Verification items for the finished model (mm, model axes). A direction names the side the tool comes from. Coordinates: 2 decimals unless noted, no trailing zeros. Order: outer loops, then holes, each group sorted by start corner. A loop starts at its lowest first (then second) coordinate and runs counter-clockwise, first axis right, second up. Notation, with made-up numbers: (80.5, 71.25) -> (114.5, 71.25) arc R25 cw to (114.5, 100.25) -> close; hole circle Ø11 at (-5, 34). An arc over 180 degrees is marked (long way). Write item = value, one per line. Start each with the question number.
1. Cross-section at B-B on y = -14. Record the cut outline in (x, z), plus the area to 3 significant figures.
2. Set-up check for faces 5 (the flat face through (-28, 0, 4)), 6 (the flat face through (-40.846, -14.79, 22.722)), 7 (the cylindrical face through (-13.654, -14.79, 21.35)), 8 (the cylindrical face through (-38.355, -14.79, 10.279)), 9 (the flat face through (-13.237, -15, 8)): record each of +Z, -Z, +X, -X, +Y, -Y from which the full face is reachable in a straight line by a thin tool's end or side.
3. Cross-section at D-D on x = -25.5. Record the cut outline in (y, z), plus the area to 3 significant figures.
4. Cross-section at C-C on x = -19. Record the cut outline in (y, z).
5. Go/stop test with flat-tipped pins: P1, Ø12, axis at y = -14.5, z = 8.5, coming from the +X side; P2, Ø1.5, axis at x = -18, z = 21, coming from the +Y side; P3, Ø1.5, axis at x = -35, y = -25.5, coming from the +Z side. Record where each tip stops, or that it passes through.
6. Release check for a two-part mould opening along X. For faces 1 (the cylindrical face through (-43.15, -14.79, 17.68)), 2 (the cylindrical face through (-17.758, -14.79, 10.556)), 3 (the flat face through (-28, -15, 0)), 4 (the cylindrical face through (-13.15, -14.79, 17.48)) record: +X half, -X half, draft (parallel to the pull), parting line (faces both ways), or undercut.
7. Cross-section at A-A on z = 17.5. Record the cut outline in (x, y), plus the area to 3 significant figures.
8. Thickness scan on line 1 along X through (y, z) = (-14, 11); line 2 along X through (y, z) = (-24.25, 9.25); line 3 along X through (y, z) = (-9.75, 4.75). Record the ranges inside material, lowest first. Write a range as from..to.
from build123d import *

# Parameters (mm, degrees)
F1_DEPTH = 30


with BuildPart() as f1:
    # F0 (on Front) → F1 (new body)
    with BuildSketch(Plane.XZ):
        with BuildLine():
            Line((-43.236702, 0), (-13.236702, 0))
            Line((-13.236702, 0), (-13.236702, 5))
            Line((-13.236702, 5), (-13.236702, 15.904253))
            Line((-13.236702, 15.904253), (-13.236702, 19.095168))
            ThreePointArc((-13.236702, 19.095168), (-13.662541, 21.381314), (-14.43662, 23.574167))
            Line((-14.43662, 23.574167), (-16.449004, 21.892771))
            ThreePointArc((-16.449004, 21.892771), (-17.85215, 10.416553), (-28.06652, 5))
            ThreePointArc((-28.06652, 5), (-28.151611, 4.99971), (-28.236702, 5))
            ThreePointArc((-28.236702, 5), (-38.451071, 10.416553), (-39.854218, 21.892771))
            Line((-39.854218, 21.892771), (-41.866602, 23.574167))
            ThreePointArc((-41.866602, 23.574167), (-42.661058, 21.304438), (-43.0826, 18.936921))
            Line((-43.0826, 18.936921), (-43.110728, 16.392998))
            Line((-43.110728, 16.392998), (-43.236702, 5))
            Line((-43.236702, 5), (-43.236702, 0))
        make_face()
        with BuildLine():
            Line((-13.236702, 19.095168), (-13.236702, 15.904253))
            ThreePointArc((-13.236702, 15.904253), (-13.151611, 17.49971), (-13.236702, 19.095168))
        make_face()
        with BuildLine():
            ThreePointArc((-43.0826, 18.936921), (-43.150694, 17.665557), (-43.110728, 16.392998))
            Line((-43.110728, 16.392998), (-43.0826, 18.936921))
        make_face()
        with BuildLine():
            ThreePointArc((-28.236702, 5), (-28.151611, 4.99971), (-28.06652, 5))
            Line((-28.06652, 5), (-28.236702, 5))
        make_face()
    extrude(amount=F1_DEPTH)


solid = f1.part
Worked out:
q1.outline = (-43.24, 0) -> (-13.24, 0) -> (-13.24, 15.9) arc R15 ccw to (-13.24, 19.1) arc R15 ccw to (-14.44, 23.57) -> (-16.45, 21.89) arc R12.5 cw to (-28.07, 5) -> (-28.24, 5) arc R12.5 cw to (-39.85, 21.89) -> (-41.87, 23.57) arc R15 ccw to (-43.08, 18.94) arc R15 ccw to (-43.11, 16.39) -> (-43.24, 5) -> close
q1.area = 306 mm²
q2.face_5 = +Z, -Z, +X, -X, +Y
q2.face_6 = +Z, +Y, -Y
q2.face_7 = +Z, +X, +Y, -Y
q2.face_8 = +Y, -Y
q2.face_9 = -Z, +X, +Y, -Y
q3.outline = (-30, 0) -> (0, 0) -> (0, 5.28) -> (-30, 5.28) -> close
q3.area = 159 mm²
q4.outline = (-30, 0) -> (0, 0) -> (0, 8.99) -> (-30, 8.99) -> close
q5.P1 = -13.24
q5.P2 = through
q5.P3 = 7.57
q6.face_1 = -X half
q6.face_2 = undercut
q6.face_3 = draft
q6.face_4 = +X half
q7.outline = (-43.15, -30) -> (-40.65, -30) -> (-40.65, 0) -> (-43.15, 0) -> close; (-15.65, -30) -> (-13.15, -30) -> (-13.15, 0) -> (-15.65, 0) -> close
q7.area = 150 mm²
q8.line_1 = -43.17..-38.83, -17.47..-13.24
q8.line_2 = -43.19..-37.54, -18.76..-13.24
q8.line_3 = -43.24..-13.24
